from build123d import *

# Parameters (mm, degrees)
BOSS_EXTRUDE1_DEPTH                             = 5
SKETCH2_R                                       = 2
CUT_EXTRUDE1_DEPTH                              = 18.720045147
CSK_FOR_M2_FLAT_HEAD_MACHINE_SCREW1_D           = 2.4
CSK_FOR_M2_FLAT_HEAD_MACHINE_SCREW1_CSINK_D     = 4.4
CSK_FOR_M2_FLAT_HEAD_MACHINE_SCREW1_CSINK_ANGLE = 90


with BuildPart() as part:
    # Sketch1 → Boss-Extrude1 (new, symmetric)
    with BuildSketch(Plane.XY):
        with BuildLine():
            Line((-6, 0), (-15, 0))
            Line((-15, 0), (-15, 8))
            Line((-15, 8), (15, 8))
            Line((15, 8), (15, 0))
            Line((15, 0), (6, 0))
            ThreePointArc((6, 0), (0, 6), (-6, 0))
        make_face()
    extrude(amount=BOSS_EXTRUDE1_DEPTH, both=True)

    # Sketch2 → Cut-Extrude1 (cut, through all)
    with BuildSketch(Plane(origin=(0, 8, 0), x_dir=(1, 0, 0), z_dir=(0, 1, 0))):
        with Locations(Location((-11, 0, 0), (0, 0, 270))):
            Circle(SKETCH2_R)
        with Locations(Location((11, 0, 0), (0, 0, 270))):
            Circle(SKETCH2_R)
    extrude(amount=-CUT_EXTRUDE1_DEPTH, mode=Mode.SUBTRACT)

    # CSK for M2 Flat Head Machine Screw1 (through all)
    with Locations(Plane(origin=(0, 8, 0), x_dir=(1, 0, 0), z_dir=(0, 1, 0))):
        with Locations((0, 0)):
            CounterSinkHole(CSK_FOR_M2_FLAT_HEAD_MACHINE_SCREW1_D / 2, CSK_FOR_M2_FLAT_HEAD_MACHINE_SCREW1_CSINK_D / 2, counter_sink_angle=CSK_FOR_M2_FLAT_HEAD_MACHINE_SCREW1_CSINK_ANGLE)


solid = part.part
Check sheet for the modelled part. Datum: model origin and axes. Units: mm. Give positions to 0.01 mm unless a question says otherwise; leave off trailing zeros. Write each loop counter-clockwise with the first axis right and the second up, starting at its lowest first coordinate (ties: lowest second). Pieces come first, ordered by that corner, then holes. Notation, with made-up numbers: (80.5, -36.75) -> (133.5, -36.75) arc R20 ccw to (133.5, -7.75) -> close; hole circle Ø3 at (-30, 82). An arc over 180 degrees is marked (long way). Write item = value, one per line.
Item 1: Sectioned sample at A-A on x = 0. Record the boundary of the cut face in (y, z), and give its area (3 significant figures).
Output:
outline = (6, -5) -> (8, -5) -> (8, -2.2) -> (7, -1.2) -> (6, -1.2) -> close; (6, 1.2) -> (7, 1.2) -> (8, 2.2) -> (8, 5) -> (6, 5) -> close
area = 14.2 mm^2
Item 2: Sectioned sample at B-B on y = 4. Record the boundary of the cut face in (x, z).
Output:
outline = (-15, -5) -> (-4.47, -5) -> (-4.47, 5) -> (-15, 5) -> close; (4.47, -5) -> (15, -5) -> (15, 5) -> (4.47, 5) -> close; hole circle Ø4 at (-11, 0); hole circle Ø4 at (11, 0)
Item 3: Scan lines: probe 1 along X at (y, z) = (6.5, -0.5); probe 2 along X at (y, z) = (2.75, -1.75); probe 3 along Z at (x, y) = (0, 7.5). Record each from-to range of solid material in increasing order. Write a range as from..to.
Output:
probe_1 = -15..-12.94, -9.06..-1.09, 1.09..9.06, 12.94..15
probe_2 = -15..-11.97, -10.03..-5.33, 5.33..10.03, 11.97..15
probe_3 = -5..-1.7, 1.7..5
Item 4: Gauge pin test, flat end, axial feed: pin 1 (2 mm diameter, centred on x = 0, z = 0, fed in from +Y). Record the tip position at first contact, or that the pin passes through.
Output:
pin_1 = through
Item 5: Sectioned sample at C-C on z = 0. Record the boundary of the cut face in (x, y).
Output:
outline = (-15, 0) -> (-13, 0) -> (-13, 8) -> (-15, 8) -> close; (-9, 0) -> (-6, 0) arc R6 cw to (-1.2, 5.88) -> (-1.2, 7) -> (-2.2, 8) -> (-9, 8) -> close; (1.2, 5.88) arc R6 cw to (6, 0) -> (9, 0) -> (9, 8) -> (2.2, 8) -> (1.2, 7) -> close; (13, 0) -> (15, 0) -> (15, 8) -> (13, 8) -> close
Item 6: Sectioned sample at D-D on y = 1.25. Record the boundary of the cut face in (x, z).
Output:
outline = (-15, -5) -> (-5.87, -5) -> (-5.87, 5) -> (-15, 5) -> close; (5.87, -5) -> (15, -5) -> (15, 5) -> (5.87, 5) -> close; hole circle Ø4 at (-11, 0); hole circle Ø4 at (11, 0)
Item 7: Release check for a two-part mould opening along Z. For faces 1 (the flat face through (-15, 4, 0)), 2 (the flat face through (0, 7, -5)), 3 (the cylindrical face through (0.26, 6.43, 1.17)) record: +Z half, -Z half, draft (parallel to the pull), parting line (faces both ways), or undercut.
Output:
face_1 = draft
face_2 = -Z half
face_3 = undercut
